```python
from build123d import *

# Parameters (mm, degrees)
SKETCH1_W           = 25
SKETCH1_H           = 40
BOSS_EXTRUDE1_DEPTH = 5
SKETCH2_R           = 2
CUT_EXTRUDE1_DEPTH  = 11.5
SKETCH3_W           = 25
SKETCH3_H           = 5
BOSS_EXTRUDE2_DEPTH = 32.25
SKETCH5_R           = 11.1
CUT_EXTRUDE2_DEPTH  = 1.5
SKETCH6_R           = 5.2
CUT_EXTRUDE3_DEPTH  = 10.5
SKETCH7_R           = 1.5
CUT_EXTRUDE4_DEPTH  = 10.5
CIRPATTERN1_COUNT   = 4
BOSS_EXTRUDE3_DEPTH = 3
BOSS_EXTRUDE4_START = 1.5
SKETCH9_R           = 11.1
SKETCH9_R_2         = 5.2
SKETCH9_R_3         = 1.5
BOSS_EXTRUDE4_DEPTH = 1.5


with BuildPart() as part:
    # Sketch1 → Boss-Extrude1 (new body)
    with BuildSketch(Plane(origin=(0, 0, 0), x_dir=(1, 0, 0), z_dir=(0, 1, 0))):
        Rectangle(SKETCH1_W, SKETCH1_H)
    extrude(amount=BOSS_EXTRUDE1_DEPTH)

    # Sketch2 → Cut-Extrude1 (cut)
    with BuildSketch(Plane(origin=(0, 5, 0), x_dir=(1, 0, 0), z_dir=(0, 1, 0))):
        with Locations(Location((0, 8, 0), (0, 0, 270))):
            Circle(SKETCH2_R)
    cut_extrude1 = extrude(amount=-CUT_EXTRUDE1_DEPTH, mode=Mode.SUBTRACT)

    # Mirror1: Cut-Extrude1 across plane
    add(cut_extrude1.mirror(Plane.XY), mode=Mode.SUBTRACT)

    # Sketch3 → Boss-Extrude2 (add)
    with BuildSketch(Plane.XZ):
        with Locations((0, 17.5)):
            Rectangle(SKETCH3_W, SKETCH3_H)
    extrude(amount=BOSS_EXTRUDE2_DEPTH)

    # Sketch5 → Cut-Extrude2 (cut)
    with BuildSketch(Plane.XY.offset(20)):
        with Locations((0, -15)):
            Circle(SKETCH5_R)
    extrude(amount=-CUT_EXTRUDE2_DEPTH, mode=Mode.SUBTRACT)

    # Sketch6 → Cut-Extrude3 (cut)
    with BuildSketch(Plane.XY.offset(18.5)):
        with Locations((0, -15)):
            Circle(SKETCH6_R)
    extrude(amount=-CUT_EXTRUDE3_DEPTH, mode=Mode.SUBTRACT)

    # Sketch7 → Cut-Extrude4 (cut)
    with BuildSketch(Plane.XY.offset(18.5)):
        with Locations((0, -7)):
            Circle(SKETCH7_R)
    cut_extrude4 = extrude(amount=-CUT_EXTRUDE4_DEPTH, mode=Mode.SUBTRACT)

    # CirPattern1: Cut-Extrude4 ×4 about axis
    cirpattern1_axis = Axis((0, -15, 0), (0, 0, 1))
    for i in range(1, CIRPATTERN1_COUNT):
        add(cut_extrude4.rotate(cirpattern1_axis, i * 360 / CIRPATTERN1_COUNT), mode=Mode.SUBTRACT)

    # Sketch8 → Boss-Extrude3 (add)
    with BuildSketch(Plane.ZY.offset(12.5)):
        Polygon((15, 0), (0, 0), (15, -11.4463543), align=None)
    boss_extrude3 = extrude(amount=-BOSS_EXTRUDE3_DEPTH)

    # Mirror2: Boss-Extrude3 across plane
    add(boss_extrude3.mirror(Plane(origin=(0, 0, 0), x_dir=(0, 0, 1), z_dir=(1, 0, 0))))

    # Sketch9 → Boss-Extrude4 (add)
    with BuildSketch(Plane.XY.offset(18.5).offset(BOSS_EXTRUDE4_START)):
        with Locations((0, -15)):
            Circle(SKETCH9_R)
        with Locations((0, -15)):
            Circle(SKETCH9_R_2, mode=Mode.SUBTRACT)
        with Locations((0, -7)):
            Circle(SKETCH9_R_3, mode=Mode.SUBTRACT)
        with Locations((-8, -15)):
            Circle(SKETCH9_R_3, mode=Mode.SUBTRACT)
        with Locations((8, -15)):
            Circle(SKETCH9_R_3, mode=Mode.SUBTRACT)
        with Locations((0, -23)):
            Circle(SKETCH9_R_3, mode=Mode.SUBTRACT)
    extrude(amount=-BOSS_EXTRUDE4_DEPTH)


solid = part.part
```
Read the model definition and answer for the solid it produces. Units are mm, in the model's axes. A direction names the side the tool comes from. Coordinates: 2 decimals unless noted, no trailing zeros. Loops run counter-clockwise (first coordinate to the right, second up) from the corner with the lowest first, then second, coordinate; pieces in that order, holes last. Notation, with made-up numbers: (72, -25.75) -> (92, -25.75) arc R20 cw to (92, -20.75) -> close; hole circle Ø2 at (50.5, 79). An arc over 180 degrees is marked (long way). Return JSON: item names as keys, results as strings.
Item 1: For a pull along X with two mould halves and no side action, classify faces 3 (the flat face through (12.5, -5, 7)), 4 (the flat face through (-9.5, -3, 11)), 5 (the flat face through (-11.021, -5.643, 7.395)) as +X half, -X half, draft (parallel to the pull), parting line (faces both ways), or undercut.
Answers:
{"face 3": "+X half", "face 4": "undercut", "face 5": "draft"}
Item 2: Find section C-C (z = 8). Determine the outline of the cut face in (x, y), plus the area to 3 significant figures.
Answers:
{"outline": "(-12.5, -6.1) -> (-9.5, -6.1) -> (-9.5, 0) -> (-2, 0) -> (-2, 5) -> (-12.5, 5) -> close; (2, 0) -> (9.5, 0) -> (9.5, -6.1) -> (12.5, -6.1) -> (12.5, 5) -> (2, 5) -> close", "area": "142 mm2"}
Item 3: Find section D-D (x = 3). Determine the outline of the cut face in (y, z).
Answers:
{"outline": "(-32.25, 15) -> (-19.25, 15) -> (-19.25, 20) -> (-32.25, 20) -> close; (-10.75, 15) -> (0, 15) -> (0, -20) -> (5, -20) -> (5, 20) -> (-10.75, 20) -> close"}
Item 4: Find section A-A (x = 0). Determine the outline of the cut face in (y, z), plus the area to 3 significant figures.
Answers:
{"outline": "(-32.25, 15) -> (-24.5, 15) -> (-24.5, 20) -> (-32.25, 20) -> close; (-21.5, 15) -> (-20.2, 15) -> (-20.2, 20) -> (-21.5, 20) -> close; (-9.8, 15) -> (-8.5, 15) -> (-8.5, 20) -> (-9.8, 20) -> close; (-5.5, 15) -> (0, 15) -> (0, 10) -> (5, 10) -> (5, 20) -> (-5.5, 20) -> close; (0, -20) -> (5, -20) -> (5, -10) -> (0, -10) -> close; (0, -6) -> (5, -6) -> (5, 6) -> (0, 6) -> close", "area": "239 mm2"}
Item 5: Flat-ended cylindrical pins translate along their axes: P1, Ø12.5, axis at x = 4.5, z = -6.5, coming from the -Y side; P2, Ø3, axis at x = -1, y = -21.5, coming from the -Z side. Find the tip coordinate at first contact, or state that the pin passes through.
Answers:
{"P1": "stops at y = 0", "P2": "stops at z = 15"}
Item 6: Find the intervals of material crossed by probe 1 along Y at (x, z) = (0, 18.45); probe 2 along X at (y, z) = (2, -8); probe 3 along X at (y, z) = (-1, 14.5), in increasing order.
Answers:
{"probe 1": "y = -32.25 to -24.5, -21.5 to -20.2, -9.8 to -8.5, -5.5 to 5", "probe 2": "x = -12.5 to -2, 2 to 12.5", "probe 3": "x = -12.5 to -9.5, 9.5 to 12.5"}
Item 7: For faces 1 (the cylindrical face through (-1.2, 2.5, -9.6)), 2 (the flat face through (0, 0, -3)), determine the directions among +Z, -Z, +X, -X, +Y, -Y from which every point of the face is accessible in a straight line to the end or side of a thin tool.
Answers:
{"face 1": "+Y, -Y", "face 2": "-Z, -Y"}
Item 8: Find section B-B (y = -24). Determine the outline of the cut face in (x, z).
Answers:
{"outline": "(-12.5, 15) -> (-1.12, 15) -> (-1.12, 20) -> (-12.5, 20) -> close; (1.12, 15) -> (12.5, 15) -> (12.5, 20) -> (1.12, 20) -> close"}
